Read the model definition and answer for the solid it produces. Units are mm, in the model's axes. A direction names the side the tool comes from. Round coordinates to 2 decimals unless told otherwise and drop trailing zeros. Order: outer loops, then holes, each group sorted by start corner. A loop starts at its lowest first (then second) coordinate and runs counter-clockwise, first axis right, second up. Notation, with made-up numbers: (14.5, 18.5) - (59.5, 18.5) arc R23 ccw to (59.5, 28.5) - close; hole circle Ø8 at (73.25, 73.5). An arc over 180 degrees is marked (long way). One line per question, with ' | ' between items. Start each with the question number.
1) The part is cut by section B-B, the plane y = 0. Give the vertices of the cut face in (x, z).
2) The mould has two halves that part along Z. Classify faces 3 (the flat face through (9, 25, 15)), 4 (the flat face through (2.5, 8, 0)), 5 (the cylindrical face through (24.61, 28.07, 8.34)), 6 (the cylindrical face through (24.61, 28.07, -5.66)): pulls with the +Z half, pulls with the -Z half, needs draft (parallel to the pull), parting line crosses it, or undercut.
3) Straight lines are drawn through the part: line 1 (X direction, y = 28, z = -7); line 2 (Z direction, x = 0.4, y = 0); line 3 (Y direction, x = 5, z = 1). For each, find the intervals that lie inside material, in ascending order. Write a range as from..to.
4) For faces 1 (the flat face through (16, 23, 0)), 2 (the flat face through (-2.5, 6, 4)), determine the directions among +Z, -Z, +X, -X, +Y, -Y from which every point of the face is accessible in a straight line to the end or side of a thin tool.
5) The part is cut by section C-C, the plane x = 22.5. Give the vertices of the cut face in (y, z).
6) The part is cut by section A-A, the plane z = 0. Give the vertices of the cut face in (x, y).
7) The part is cut by section D-D, the plane z = -5.75. Give the vertices of the cut face in (x, y).
8) Flat-ended cylindrical pins translate along their axes: pin 1 (9 mm diameter, centred on y = 4, z = 0.5, fed in from +X); pin 2 (14 mm diameter, centred on x = 18, z = 6, fed in from -Y). Find the tip coordinate at first contact, or state that the pin passes through.
from build123d import *

# Parameters (mm, degrees)
BOSS_EXTRUDE2_DEPTH      = 2.5
BOSS_EXTRUDE3_DEPTH      = 30
BOSS_EXTRUDE3_DEPTH_BACK = 2.5
SKETCH2_R                = 2.4999999999999982
CUT_EXTRUDE1_DEPTH       = 12.999999999999984
FILLET1_R                = 4


with BuildPart() as part:
    # Sketch1 → Boss-Extrude2 (new, symmetric)
    with BuildSketch(Plane(origin=(0, 0, 0), x_dir=(0, 0, -1), z_dir=(1, 0, 0))):
        with BuildLine():
            Line((1.22e-15, -17), (0, -6.999999999999999))
            ThreePointArc((-1.29e-15, -6.999999999999999), (-6.999999999999999, 8.6e-16), (4.3e-16, 6.999999999999999))
            Line((0, 7), (1.22e-15, 23))
            Line((1.22e-15, 23), (-15, 22.999999999999996))
            Line((-14.999999999999998, 22.999999999999996), (-14.999999999999993, -17))
            Line((-14.999999999999993, -17), (1.78e-15, -17))
        make_face()
        with BuildLine():
            ThreePointArc((6.999999999999999, -1.71e-15), (4.949747468305831, -4.949747468305834), (-1.29e-15, -6.999999999999999))
            Line((0, -6.999999999999999), (1.22e-15, -17))
            Line((1.22e-15, -17), (15, -17))
            Line((15, -17), (15, 23))
            Line((15, 23), (1.22e-15, 23))
            Line((1.22e-15, 23), (0, 7))
            ThreePointArc((4.3e-16, 6.999999999999999), (4.949747468305833, 4.949747468305832), (6.999999999999999, 0))
        make_face()
    extrude(amount=BOSS_EXTRUDE2_DEPTH, both=True)

    # Sketch1_7 → Boss-Extrude3 (add, two sides: drawn at the far end of the back side and taken through both)
    with BuildSketch(Plane(origin=(0, 0, 0), x_dir=(0, 0, -1), z_dir=(1, 0, 0)).offset(-BOSS_EXTRUDE3_DEPTH_BACK)):
        Polygon((-15, 22.999999999999996), (1.22e-15, 23), (-1.73e-15, 33), (-15, 33), align=None)
        Polygon((-1.73e-15, 33), (1.22e-15, 23), (15, 23), (15, 33.00000000000001), align=None)
    extrude(amount=BOSS_EXTRUDE3_DEPTH + BOSS_EXTRUDE3_DEPTH_BACK)

    # Sketch2 → Cut-Extrude1 (cut)
    with BuildSketch(Plane(origin=(0, 33, 0), x_dir=(1, 0, 0), z_dir=(0, 1, 0))):
        with Locations(Location((22.5, -7.000000000000001, 0), (0, 0, 270))):
            Circle(SKETCH2_R)
        with Locations(Location((22.5, 6.999999999999999, 0), (0, 0, 270))):
            Circle(SKETCH2_R)
    extrude(amount=-CUT_EXTRUDE1_DEPTH, mode=Mode.SUBTRACT)

    # Fillet1
    fillet1_edges = [part.edges().sort_by_distance(p)[0] for p in [
        (-2.5, 33, 0),
    ]]
    fillet(fillet1_edges, radius=FILLET1_R)


solid = part.part
Values:
1) outline: (-2.5, -15) - (2.5, -15) - (2.5, -7) - (-2.5, -7) - close; (-2.5, 7) - (2.5, 7) - (2.5, 15) - (-2.5, 15) - close
2) face 3: pulls with the +Z half | face 4: needs draft | face 5: undercut | face 6: undercut
3) line 1: x = -2.5..20, 25..30 | line 2: z = -15..-7, 7..15 | line 3: y = 23..33
4) face 1: +Z, -Z, +X, -Y | face 2: +Z, -Z, -X, +Y, -Y
5) outline: (23, -15) - (33, -15) - (33, -9.5) - (23, -9.5) - close; (23, -4.5) - (33, -4.5) - (33, 4.5) - (23, 4.5) - close; (23, 9.5) - (33, 9.5) - (33, 15) - (23, 15) - close
6) outline: (-2.5, -17) - (2.5, -17) - (2.5, -7) - (-2.5, -7) - close; (-2.5, 7) - (2.5, 7) - (2.5, 23) - (30, 23) - (30, 33) - (1.5, 33) arc R4 ccw to (-2.5, 29) - close
7) outline: (-2.5, -17) - (2.5, -17) - (2.5, -3.99) - (-2.5, -3.99) - close; (-2.5, 3.99) - (2.5, 3.99) - (2.5, 23) - (20.33, 23) - (20.33, 33) - (1.5, 33) arc R4 ccw to (-2.5, 29) - close; (24.67, 23) - (30, 23) - (30, 33) - (24.67, 33) - close
8) pin 1: stops at x = 2.5 | pin 2: stops at y = 23
